```python
from build123d import *

# Parameters (mm, degrees)
F0_R     = 1.5
F1_DEPTH = 3


with BuildPart() as f1:
    # F0 (on Top) → F1 (new body)
    with BuildSketch(Plane.XY):
        with BuildLine():
            Line((7.5, 3), (0, 3))
            Line((0, 3), (-7.5, 3))
            ThreePointArc((-7.5, 3), (-5.37868, 2.12132), (-4.5, 0))
            ThreePointArc((-4.5, 0), (-5.37868, -2.12132), (-7.5, -3))
            Line((-7.5, -3), (0, -3))
            Line((0, -3), (7.5, -3))
            ThreePointArc((7.5, -3), (10.5, 0), (7.5, 3))
        make_face()
        with BuildLine():
            ThreePointArc((-1, -1.5), (-2.5, 0), (-1, 1.5))
            Line((-1, 1.5), (7.5, 1.5))
            ThreePointArc((7.5, 1.5), (8.56066, 1.06066), (9, 0))
            ThreePointArc((9, 0), (8.56066, -1.06066), (7.5, -1.5))
            Line((7.5, -1.5), (-1, -1.5))
        make_face(mode=Mode.SUBTRACT)
        with BuildLine():
            ThreePointArc((-4.5, 0), (-5.37868, 2.12132), (-7.5, 3))
            ThreePointArc((-7.5, 3), (-10.5, 0), (-7.5, -3))
            ThreePointArc((-7.5, -3), (-5.37868, -2.12132), (-4.5, 0))
        make_face()
        with Locations((-7.5, 0)):
            Circle(F0_R, mode=Mode.SUBTRACT)
    extrude(amount=F1_DEPTH)


solid = f1.part
```
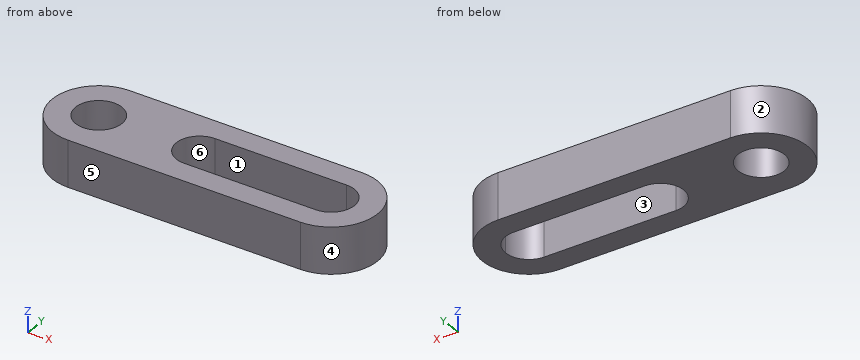
Here's how the part is built. I have some questions about the finished solid (model axes, mm). Face numbers are marked on the shaded views. A direction names the side the tool comes from. Give positions to 0.01 mm unless a question says otherwise; leave off trailing zeros. Loops run counter-clockwise (first coordinate to the right, second up) from the corner with the lowest first, then second, coordinate; pieces in that order, holes last. Notation, with made-up numbers: M 37.25,26 L 54.25,26 A26 ccw 54.25,49 Z; hole C -21.5,19 d9. An arc over 180 degrees is marked long. Use one line per item in the form item = value. Start each with the question number.
Q1. If we section it at C-C (x = -7.75): Write out the boundary of the cut face in (y, z).
Q2. Which directions (+Z, -Z, +X, -X, +Y, -Y) give clear straight access to the entire face, cutting with the end or side of a thin tool? Please do the marked faces 5 and 6.
Q3. If we section it at B-B (y = 0.95): Write out the boundary of the cut face in (x, z), then the cut area to 3 significant figures.
Q4. If we section it at A-A (z = 2.4): Write out the boundary of the cut face in (x, y), then the cut area to 3 significant figures.
Q5. Thinking about a two-plate mould opening in X: for the marked faces 1, 2, 3 and 4, which applies, +X half, -X half, draft (parallel to the pull), parting line (faces both ways), or undercut?
Q6. If we section it at D-D (y = -0.9): Write out the boundary of the cut face in (x, z).
Q7. I need wall thicknesses on line 1 along Y through (x, z) = (2, 2.6); line 2 along X through (y, z) = (-0.4, 0.25); line 3 along X through (y, z) = (-0.6, 1.1). Which ranges of each line are inside material? Lowest first, please.
Taken from the geometry:
q1.outline = M -2.99,0 L -1.48,0 L -1.48,3 L -2.99,3 Z; M 1.48,0 L 2.99,0 L 2.99,3 L 1.48,3 Z
q2.face_5 = +Z, -Z, +X, -X, -Y
q2.face_6 = +Z, -Z
q3.outline = M -10.35,0 L -8.66,0 L -8.66,3 L -10.35,3 Z; M -6.34,0 L -2.16,0 L -2.16,3 L -6.34,3 Z; M 8.66,0 L 10.35,0 L 10.35,3 L 8.66,3 Z
q3.area = 22.6 mm^2
q4.outline = M -7.5,-3 L 7.5,-3 A3 ccw 7.5,3 L -7.5,3 A3 ccw Z; hole C -7.5,0 d3; hole M -1,-1.5 L 7.5,-1.5 A1.5 ccw 9,0 A1.5 ccw 7.5,1.5 L -1,1.5 A1.5 ccw Z
q4.area = 78.6 mm^2
q5.face_1 = undercut
q5.face_2 = -X half
q5.face_3 = undercut
q5.face_4 = +X half
q6.outline = M -10.36,0 L -8.7,0 L -8.7,3 L -10.36,3 Z; M -6.3,0 L -2.2,0 L -2.2,3 L -6.3,3 Z; M 8.7,0 L 10.36,0 L 10.36,3 L 8.7,3 Z
q7.line_1 = -3 to -1.5, 1.5 to 3
q7.line_2 = -10.47 to -8.95, -6.05 to -2.45, 8.95 to 10.47
q7.line_3 = -10.44 to -8.87, -6.13 to -2.37, 8.87 to 10.44
